For this review, take the finished solid that the model builds, in its own axes (mm). A direction names the side the tool comes from. Coordinates: 2 decimals unless noted, no trailing zeros. Write each loop counter-clockwise with the first axis right and the second up, starting at its lowest first coordinate (ties: lowest second). Pieces come first, ordered by that corner, then holes.
1) We need section C-C on y = 6.5. Write out the cut boundary in (x, z).
2) Insertion check: P1, Ø1, axis at y = -20, z = 76.5, coming from the +X side; P2, Ø3, axis at x = -24, y = 21.5, coming from the -Z side. Each pin has a flat end and moves straight along its axis. Give the tip position at first contact, or say it passes through.
3) We need section A-A on x = -4.5. Write out the cut boundary in (y, z).
4) To check wall thickness, follow line 1 along Y through (x, z) = (-46.5, 35.5); line 2 along X through (y, z) = (26, 89.5); line 3 along Z through (x, y) = (45, -25.5). State the ranges of each line that lie inside material, in increasing order.
5) Mouldability with a two-part tool opening along Y and no side actions: class faces 1 (the face through (-1, -55, 64)), 2 (the face through (-55, -1, 64)), 3 (the face through (2, 1, 110)) as pulls with the +Y half, pulls with the -Y half, needs draft (parallel to the pull), parting line crosses it, or undercut.
6) We need section B-B on z = 35.5. Write out the cut boundary in (x, y), then the cut area to 3 significant figures.
7) For faces 4 (the face through (3, -50, 54)), 5 (the face through (-53, 0, 0)), list the 3-axis set-ups (+Z, -Z, +X, -X, +Y, -Y) from which the entire face can be reached by the end or side of a thin tool; tool diameter is ignored.
from build123d import *

# Parameters (mm, degrees)
SKETCH_1_W               = 110
SKETCH_1_H               = 110
EXTRUDE_1_DEPTH          = 130
SKETCH_2_W               = 100
SKETCH_2_H               = 100
CUT_EXTRUDE_1_DEPTH      = 110
CUT_EXTRUDE_2_DEPTH      = 179.955301682
CUT_EXTRUDE_2_DEPTH_BACK = 10


with BuildPart() as part:
    # 草图1 → 凸台-拉伸1 (new body)
    with BuildSketch(Plane.XY):
        Rectangle(SKETCH_1_W, SKETCH_1_H)
    extrude(amount=EXTRUDE_1_DEPTH)

    # 草图2 → 切除-拉伸1 (cut)
    with BuildSketch(Plane(origin=(0, 0, 0), x_dir=(-1, 0, 0), z_dir=(0, 0, -1))):
        Rectangle(SKETCH_2_W, SKETCH_2_H)
    extrude(amount=-CUT_EXTRUDE_1_DEPTH, mode=Mode.SUBTRACT)

    # 草图3 → 切除-拉伸2 (cut, two sides: drawn at the far end of the back side and taken through both)
    with BuildSketch(Plane(origin=(55, 0, 0), x_dir=(0, 0, -1), z_dir=(1, 0, 0)).offset(-CUT_EXTRUDE_2_DEPTH_BACK)):
        Polygon((344.215499341, 50), (0, 50), (-110, 50), (-110, -50), (0, -50), (344.215499341, -50), (1032.646498024, -50), (1032.646498024, 50), align=None)
    extrude(amount=CUT_EXTRUDE_2_DEPTH + CUT_EXTRUDE_2_DEPTH_BACK, mode=Mode.SUBTRACT)


solid = part.part
Result:
1. outline: (-55, 0) - (-50, 0) - (-50, 110) - (55, 110) - (55, 130) - (-55, 130) - close
2. P1: stops at x = -50
2. P2: stops at z = 110
3. outline: (-55, 0) - (-50, 0) - (-50, 110) - (50, 110) - (50, 0) - (55, 0) - (55, 130) - (-55, 130) - close
4. line 1: y = -55 to -50, 50 to 55
4. line 2: x = -55 to -50
4. line 3: z = 110 to 130
5. face 1: pulls with the -Y half
5. face 2: needs draft
5. face 3: undercut
6. outline: (-55, -55) - (55, -55) - (55, -50) - (-50, -50) - (-50, 50) - (55, 50) - (55, 55) - (-55, 55) - close
6. area: 1,600 mm2
7. face 4: -Z, +X
7. face 5: -Z, +X, -X, +Y, -Y
